Can you work these out from the model? Positions are in its coordinate system, mm. A direction names the side the tool comes from. Give positions to 0.01 mm unless a question says otherwise; leave off trailing zeros. Write each loop counter-clockwise with the first axis right and the second up, starting at its lowest first coordinate (ties: lowest second). Pieces come first, ordered by that corner, then holes. Notation, with made-up numbers: (41, 74.25) -> (48, 74.25) arc R6 ccw to (48, 79.25) -> close; hole circle Ø1 at (5, 72.25). An arc over 180 degrees is marked (long way). Answer as CSV lines item,"result". Start each with the question number.
1. If we mould it in two halves opening along Y, with no side actions, what happens to faces 4 (the face through (26, 9, 7)), 5 (the face through (31.5, 2, 5)), 6 (the face through (47.14, 1.4, 5.07))? For each: pulls with the +Y half, pulls with the -Y half, needs draft (parallel to the pull), parting line crosses it, or undercut.
2. If we section it at A-A on x = 14.5: Write out the boundary of the cut face in (y, z).
3. I need wall thicknesses on line 1 (Y direction, x = 14.5, z = 3.25); line 2 (Y direction, x = 14.5, z = 6); line 3 (Y direction, x = 42.5, z = 7.75). Which ranges of each line are inside material? Lowest first, please. Write a range as [from, to].
4. I'm going to push flat-ended pins straight in: P1, Ø1, axis at x = 47.5, z = 7.5, coming from the +Y side; P2, Ø1, axis at x = 55.5, z = 5.5, coming from the +Y side; P3, Ø2.5, axis at x = 53.5, z = 4, coming from the -Y side; P4, Ø5, axis at x = 16.5, y = 36.5, coming from the -Z side. Where does each tip first touch, or does it pass through?
5. If we section it at C-C on x = 42.5: Write out the boundary of the cut face in (y, z), plus the area to 3 significant figures.
6. If we section it at B-B on y = 6.5: Write out the boundary of the cut face in (x, z), plus the area to 3 significant figures.
7. If we section it at D-D on y = 30.5: Write out the boundary of the cut face in (x, z).
8. On a 3-axis mill with a long thin cutter (end or side, diameter ignored), from which of +Z, -Z, +X, -X, +Y, -Y can I reach the whole of each face in a straight line? I mean faces 1 (the face through (55, 84, 5)), 2 (the face through (25.5, 2, 5)), 3 (the face through (43, 32, 7)). Say none if no direction works.
```python
from build123d import *

# Parameters (mm, degrees)
BOX014_W               = 19
BOX014_H               = 62
BOX014_DEPTH           = 10
BOX013_W               = 34
BOX013_H               = 75
BOX013_DEPTH           = 10
BOX002_W               = 9
BOX002_H               = 9
BOX002_DEPTH           = 10
BOX003_W               = 9
BOX003_H               = 19
BOX003_DEPTH           = 10
BOX004_W               = 9
BOX004_H               = 9
BOX004_DEPTH           = 10
BOX005_W               = 2
BOX005_H               = 6
BOX005_DEPTH           = 10
BOX006_W               = 2
BOX006_H               = 8
BOX006_DEPTH           = 10
BOX007_W               = 2
BOX007_H               = 6
BOX007_DEPTH           = 10
BOX008_W               = 2
BOX008_H               = 6
BOX008_DEPTH           = 10
BOX009_W               = 2
BOX009_H               = 6
BOX009_DEPTH           = 10
BOX010_W               = 2
BOX010_H               = 8
BOX010_DEPTH           = 10
CYLINDER_R             = 4
CYLINDER_DEPTH         = 10
CYLINDER002_R          = 4
CYLINDER002_DEPTH      = 10
CYLINDER001_R          = 4
CYLINDER001_DEPTH      = 10
CYLINDER003_R          = 4
CYLINDER003_DEPTH      = 10
BOX011_W               = 3
BOX011_H               = 6
BOX011_DEPTH           = 10
BOX011_PLACEMENT_ANGLE = 90
BOX012_W               = 3
BOX012_H               = 6
BOX012_DEPTH           = 10
BOX012_PLACEMENT_ANGLE = 90
BOX001_W               = 9
BOX001_H               = 19
BOX001_DEPTH           = 10
BOX_W                  = 57
BOX_H                  = 107
BOX_DEPTH              = 10
FILLET_R               = 3
FILLET001_R            = 4


with BuildPart() as cube014:
    # Box014 → Box014 (new body)
    with BuildSketch(Plane(origin=(33, 32, 5), x_dir=(1, 0, 0), z_dir=(0, 0, 1))):
        with Locations((9.5, 31)):
            Rectangle(BOX014_W, BOX014_H)
    extrude(amount=BOX014_DEPTH)


with BuildPart() as fusion001:
    # Box013 → Box013 (new body)
    with BuildSketch(Plane(origin=(0, 9, 5), x_dir=(1, 0, 0), z_dir=(0, 0, 1))):
        with Locations((17, 37.5)):
            Rectangle(BOX013_W, BOX013_H)
    extrude(amount=BOX013_DEPTH)

    # Fusion001: union Cube014
    add(cube014.part)


with BuildPart() as cube002:
    # Box002 → Box002 (new body)
    with BuildSketch(Plane.XY):
        with Locations((4.5, 4.5)):
            Rectangle(BOX002_W, BOX002_H)
    extrude(amount=BOX002_DEPTH)


with BuildPart() as cube003:
    # Box003 → Box003 (new body)
    with BuildSketch(Plane(origin=(0, 89, 0), x_dir=(1, 0, 0), z_dir=(0, 0, 1))):
        with Locations((4.5, 9.5)):
            Rectangle(BOX003_W, BOX003_H)
    extrude(amount=BOX003_DEPTH)


with BuildPart() as cube004:
    # Box004 → Box004 (new body)
    with BuildSketch(Plane(origin=(48, 99, 0), x_dir=(1, 0, 0), z_dir=(0, 0, 1))):
        with Locations((4.5, 4.5)):
            Rectangle(BOX004_W, BOX004_H)
    extrude(amount=BOX004_DEPTH)


with BuildPart() as cube005:
    # Box005 → Box005 (new body)
    with BuildSketch(Plane(origin=(0, 51, 0), x_dir=(1, 0, 0), z_dir=(0, 0, 1))):
        with Locations((1, 3)):
            Rectangle(BOX005_W, BOX005_H)
    extrude(amount=BOX005_DEPTH)


with BuildPart() as cube006:
    # Box006 → Box006 (new body)
    with BuildSketch(Plane(origin=(0, 81, 0), x_dir=(1, 0, 0), z_dir=(0, 0, 1))):
        with Locations((1, 4)):
            Rectangle(BOX006_W, BOX006_H)
    extrude(amount=BOX006_DEPTH)


with BuildPart() as cube007:
    # Box007 → Box007 (new body)
    with BuildSketch(Plane(origin=(0, 21, 0), x_dir=(1, 0, 0), z_dir=(0, 0, 1))):
        with Locations((1, 3)):
            Rectangle(BOX007_W, BOX007_H)
    extrude(amount=BOX007_DEPTH)


with BuildPart() as cube008:
    # Box008 → Box008 (new body)
    with BuildSketch(Plane(origin=(55, 51, 0), x_dir=(1, 0, 0), z_dir=(0, 0, 1))):
        with Locations((1, 3)):
            Rectangle(BOX008_W, BOX008_H)
    extrude(amount=BOX008_DEPTH)


with BuildPart() as cube009:
    # Box009 → Box009 (new body)
    with BuildSketch(Plane(origin=(55, 81, 0), x_dir=(1, 0, 0), z_dir=(0, 0, 1))):
        with Locations((1, 3)):
            Rectangle(BOX009_W, BOX009_H)
    extrude(amount=BOX009_DEPTH)


with BuildPart() as cube010:
    # Box010 → Box010 (new body)
    with BuildSketch(Plane(origin=(55, 19, 0), x_dir=(1, 0, 0), z_dir=(0, 0, 1))):
        with Locations((1, 4)):
            Rectangle(BOX010_W, BOX010_H)
    extrude(amount=BOX010_DEPTH)


with BuildPart() as cylinder:
    # Cylinder → Cylinder (new body)
    with BuildSketch(Plane(origin=(14.5, 6.5, 0), x_dir=(1, 0, 0), z_dir=(0, 0, 1))):
        Circle(CYLINDER_R)
    extrude(amount=CYLINDER_DEPTH)


with BuildPart() as cylinder002:
    # Cylinder002 → Cylinder002 (new body)
    with BuildSketch(Plane(origin=(42.5, 101.5, 0), x_dir=(1, 0, 0), z_dir=(0, 0, 1))):
        Circle(CYLINDER002_R)
    extrude(amount=CYLINDER002_DEPTH)


with BuildPart() as cylinder001:
    # Cylinder001 → Cylinder001 (new body)
    with BuildSketch(Plane(origin=(42.5, 6.5, 0), x_dir=(1, 0, 0), z_dir=(0, 0, 1))):
        Circle(CYLINDER001_R)
    extrude(amount=CYLINDER001_DEPTH)


with BuildPart() as cylinder003:
    # Cylinder003 → Cylinder003 (new body)
    with BuildSketch(Plane(origin=(14.5, 101.5, 0), x_dir=(1, 0, 0), z_dir=(0, 0, 1))):
        Circle(CYLINDER003_R)
    extrude(amount=CYLINDER003_DEPTH)


with BuildPart() as cube011:
    # Box011 → Box011 (new body)
    with BuildSketch(Plane.XY):
        with Locations((1.5, 3)):
            Rectangle(BOX011_W, BOX011_H)
    extrude(amount=BOX011_DEPTH)


with BuildPart() as cube011_1:
    # Box011 placement: moved
    add(cube011.part.moved(Location((31.5, 0, 0))).rotate(Axis((31.5, 0, 0), (0, 0, 1)), BOX011_PLACEMENT_ANGLE))


with BuildPart() as cube012:
    # Box012 → Box012 (new body)
    with BuildSketch(Plane.XY):
        with Locations((1.5, 3)):
            Rectangle(BOX012_W, BOX012_H)
    extrude(amount=BOX012_DEPTH)


with BuildPart() as cube012_1:
    # Box012 placement: moved
    add(cube012.part.moved(Location((31.5, 105, 0))).rotate(Axis((31.5, 105, 0), (0, 0, 1)), BOX012_PLACEMENT_ANGLE))


with BuildPart() as fusion:
    # Box001 → Box001 (new body)
    with BuildSketch(Plane(origin=(48, 0, 0), x_dir=(1, 0, 0), z_dir=(0, 0, 1))):
        with Locations((4.5, 9.5)):
            Rectangle(BOX001_W, BOX001_H)
    extrude(amount=BOX001_DEPTH)

    # Fusion: union Cube002, Cube003, Cube004, Cube005, Cube006, Cube007, Cube008, Cube009, Cube010, Cylinder, Cylinder002, Cylinder001, Cylinder003, Cube011, Cube012
    add(cube002.part)
    add(cube003.part)
    add(cube004.part)
    add(cube005.part)
    add(cube006.part)
    add(cube007.part)
    add(cube008.part)
    add(cube009.part)
    add(cube010.part)
    add(cylinder.part)
    add(cylinder002.part)
    add(cylinder001.part)
    add(cylinder003.part)
    add(cube011_1.part)
    add(cube012_1.part)


with BuildPart() as cut001:
    # Box → Box (new body)
    with BuildSketch(Plane(origin=(0, 0.5, 0), x_dir=(1, 0, 0), z_dir=(0, 0, 1))):
        with Locations((28.5, 53.5)):
            Rectangle(BOX_W, BOX_H)
    extrude(amount=BOX_DEPTH)

    # Cut: cut Fusion
    add(fusion.part, mode=Mode.SUBTRACT)

    # Fillet
    fillet_edges = [cut001.edges().sort_by_distance(p)[0] for p in [
        (9, 107.5, 5),
        (48, 107.5, 5),
        (57, 99, 5),
        (48, 0.5, 5),
        (9, 0.5, 5),
        (0, 9, 5),
    ]]
    fillet(fillet_edges, radius=FILLET_R)

    # Fillet001
    fillet001_edges = [cut001.edges().sort_by_distance(p)[0] for p in [
        (9, 89, 5),
        (48, 99, 5),
        (9, 9, 5),
        (48, 19, 5),
    ]]
    fillet(fillet001_edges, radius=FILLET001_R)

    # Cut001: cut Fusion001
    add(fusion001.part, mode=Mode.SUBTRACT)


solid = cut001.part
```
Computed values:
1,face 4,"undercut"
1,face 5,"needs draft"
1,face 6,"pulls with the -Y half"
2,outline,"(0.5, 0) -> (2.5, 0) -> (2.5, 10) -> (0.5, 10) -> close; (10.5, 0) -> (97.5, 0) -> (97.5, 10) -> (84, 10) -> (84, 5) -> (10.5, 5) -> close; (105.5, 0) -> (107.5, 0) -> (107.5, 10) -> (105.5, 10) -> close"
3,line 1,"y = [0.5, 2.5], [10.5, 97.5], [105.5, 107.5]"
3,line 2,"y = [0.5, 2.5], [84, 97.5], [105.5, 107.5]"
3,line 3,"y = [0.5, 2.5], [10.5, 32], [94, 97.5], [105.5, 107.5]"
4,P1,"stops at y = 106.74"
4,P2,"stops at y = 98.83"
4,P3,"stops at y = 19"
4,P4,"stops at z = 0"
5,outline,"(0.5, 0) -> (2.5, 0) -> (2.5, 10) -> (0.5, 10) -> close; (10.5, 0) -> (97.5, 0) -> (97.5, 10) -> (94, 10) -> (94, 5) -> (32, 5) -> (32, 10) -> (10.5, 10) -> close; (105.5, 0) -> (107.5, 0) -> (107.5, 10) -> (105.5, 10) -> close"
5,area,"600 mm2"
6,outline,"(8.71, 0) -> (10.5, 0) -> (10.5, 10) -> (8.71, 10) -> close; (18.5, 0) -> (38.5, 0) -> (38.5, 10) -> (18.5, 10) -> close; (46.5, 0) -> (48, 0) -> (48, 10) -> (46.5, 10) -> close"
6,area,"233 mm2"
7,outline,"(0, 0) -> (57, 0) -> (57, 10) -> (34, 10) -> (34, 5) -> (0, 5) -> close"
8,face 1,"+Z, -Z, +X"
8,face 2,"+Z, -Z, -Y"
8,face 3,"+Z, -X"
